Source: CAD feature listing. Evaluate the final solid. Frame: model axes, mm. Give positions to 0.01 mm unless a question says otherwise; leave off trailing zeros. Order: outer loops, then holes, each group sorted by start corner. A loop starts at its lowest first (then second) coordinate and runs counter-clockwise, first axis right, second up.
```python
from build123d import *

# Parameters (mm, degrees)
DODANIE_WYCI_GNI_CIE1_DEPTH                         = 1400
POG_BIENIE_WALCOWE_POD_M6_WKR_T_Z_BEM_W_D           = 6.6
POG_BIENIE_WALCOWE_POD_M6_WKR_T_Z_BEM_W_CBORE_D     = 11
POG_BIENIE_WALCOWE_POD_M6_WKR_T_Z_BEM_W_CBORE_DEPTH = 6.4
SZYK_LINIOWY1_COUNT                                 = 23
SZYK_LINIOWY1_PITCH                                 = 60


with BuildPart() as part:
    # Szkic1 → Dodanie-wyciągnięcie1 (new body)
    with BuildSketch(Plane.XY):
        Polygon((10, 0), (-10, 0), (-10, 4), (-6, 8), (-6, 10), (-10, 14), (-10, 15), (-7.5, 17.5), (0, 17.5), (7.5, 17.5), (10, 15), (10, 14), (6, 10), (6, 8), (10, 4), align=None)
    extrude(amount=DODANIE_WYCI_GNI_CIE1_DEPTH)

    # Pogłębienie walcowe pod M6 Wkręt z łbem walcowym z gniazdem sześciokątnym1 (through all)
    with Locations(Plane(origin=(0, 17.5, 0), x_dir=(1, 0, 0), z_dir=(0, 1, 0))):
        with Locations((0, -1380)):
            pog_bienie_walcowe_pod_m6_wkr_t_z_bem_w = CounterBoreHole(POG_BIENIE_WALCOWE_POD_M6_WKR_T_Z_BEM_W_D / 2, POG_BIENIE_WALCOWE_POD_M6_WKR_T_Z_BEM_W_CBORE_D / 2, POG_BIENIE_WALCOWE_POD_M6_WKR_T_Z_BEM_W_CBORE_DEPTH)

    # Szyk liniowy1: Pogłębienie walcowe pod M6 Wkręt z łbem walcowym z gniazdem sześciokątnym1 ×23
    with Locations(*[(0, 0, -i * SZYK_LINIOWY1_PITCH) for i in range(1, SZYK_LINIOWY1_COUNT)]):
        add(pog_bienie_walcowe_pod_m6_wkr_t_z_bem_w, mode=Mode.SUBTRACT)


solid = part.part
```
1) Pin query (flat end, axial travel): pin 1 (3.5 mm diameter, centred on x = -2.5, z = 1198, fed in from +Y); pin 2 (3 mm diameter, centred on x = 8, z = 1073, fed in from -Y); pin 3 (5.5 mm diameter, centred on x = 0, z = 360, fed in from -Y); pin 4 (0.6 mm diameter, centred on y = 9, z = 849.5, fed in from -X). Return the tip coordinate at first contact, or that it passes through.
Report:
pin 1: stops at y = 11.1
pin 2: stops at y = 0
pin 3: passes through
pin 4: stops at x = -6
2) Material intervals for L1, parallel to X at y = 6.5, z = 120.5; L2, parallel to X at y = 6.75, z = 1080; L3, parallel to Y at x = -8, z = 845.5, sorted ascending.
Report:
L1: x = -7.5 to -3.26, 3.26 to 7.5
L2: x = -7.25 to -3.3, 3.3 to 7.25
L3: y = 0 to 6, 12 to 17
3) Section query A-A, the plane z = 265. Return the cut outline in (x, y), and give its area (3 significant figures).
Report:
outline: (-10, 0) - (10, 0) - (10, 4) - (6, 8) - (6, 10) - (10, 14) - (10, 15) - (7.5, 17.5) - (-7.5, 17.5) - (-10, 15) - (-10, 14) - (-6, 10) - (-6, 8) - (-10, 4) - close
area: 296 mm2
